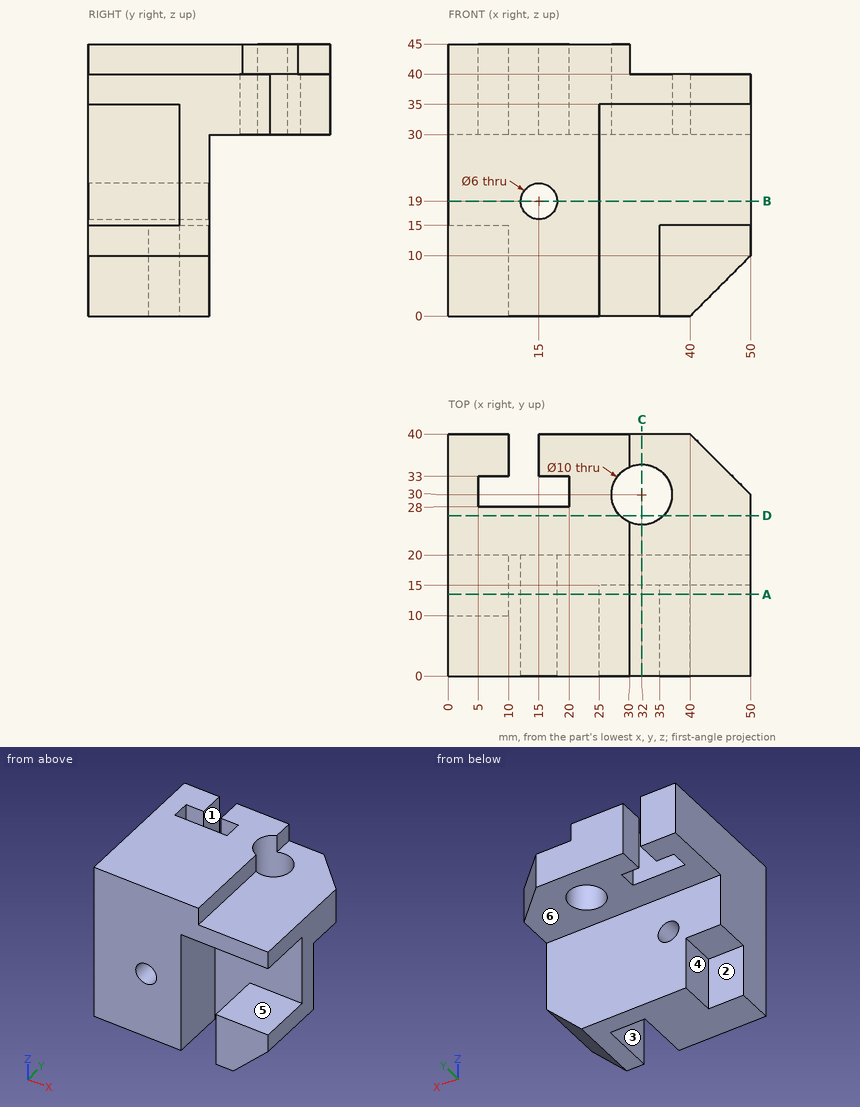
Geometry check sheet. Reference: drawing and pictorial views, mm from the part's lowest x, y, z. A direction names the side the tool comes from. Give positions to 0.01 mm unless a question says otherwise; leave off trailing zeros. Order: outer loops, then holes, each group sorted by start corner. A loop starts at its lowest first (then second) coordinate and runs counter-clockwise, first axis right, second up. Notation, with made-up numbers: M 59.25,-35.75 L 118.25,-35.75 A19 cw 118.25,-10.75 Z; hole C 65,-11 d6. An arc over 180 degrees is marked long. Answer in a Markdown table with one row per item. Add a question column.
Item 1: Mould release check, pull along Z, two halves, no side actions. Record for the marked faces 4, 5 and 6: released by +Z, released by -Z, zero draft, split by the parting line, or undercut.
Item 2: Scan lines: probe 1 along X at (y, z) = (5, 19); probe 2 along X at (y, z) = (30, 37.5); probe 3 along X at (y, z) = (30, 40.75). Record each from-to range of solid material in increasing order. Write a range as from..to.
Item 3: Section check B-B, the plane z = 19. Enter the section's corners in (x, y), and give its area (3 significant figures).
Item 4: Tool access check on the marked faces 1, 2 and 3. Record the directions out of +Z, -Z, +X, -X, +Y, -Y that give a thin tool (end or side, any length) a straight path to the whole face; none if there is none.
Item 5: Section check C-C, the plane x = 32. Enter the section's corners in (y, z), and give its area (3 significant figures).
Item 6: Gauge pin test, flat ends, axial feed: pin 1 (5 mm diameter, centred on x = 4, y = 15.5, fed in from -Z); pin 2 (1 mm diameter, centred on x = 11.5, z = 26.5, fed in from +Y); pin 3 (10 mm diameter, centred on x = 42, y = 29.5, fed in from +Z). Record the tip position at first contact, or that the pin passes through.
Item 7: Section check A-A, the plane y = 13.5. Enter the section's corners in (x, z).
Item 8: Section check D-D, the plane y = 26.5. Enter the section's corners in (x, z), and give its area (3 significant figures).
Filled sheet:
| question | item | result |
|---|---|---|
| 1 | face 4 | zero draft |
| 1 | face 5 | undercut |
| 1 | face 6 | released by -Z |
| 2 | probe 1 | x = 0..12, 18..25 |
| 2 | probe 2 | x = 0..5, 20..27, 37..50 |
| 2 | probe 3 | x = 0..5, 20..27 |
| 3 | outline | M 0,0 L 12,0 L 12,20 L 0,20 Z; M 18,0 L 25,0 L 25,15 L 50,15 L 50,20 L 18,20 Z |
| 3 | area | 505 mm^2 |
| 4 | face 1 | +Z, -Z, +Y |
| 4 | face 2 | -Z, -X, +Y |
| 4 | face 3 | -Z, -Y |
| 5 | outline | M 0,35 L 15,35 L 15,0 L 20,0 L 20,30 L 25,30 L 25,40 L 0,40 Z; M 35,30 L 40,30 L 40,40 L 35,40 Z |
| 5 | area | 375 mm^2 |
| 6 | pin 1 | stops at z = 15 |
| 6 | pin 2 | stops at y = 20 |
| 6 | pin 3 | stops at z = 40 |
| 7 | outline | M 0,15 L 10,15 L 10,0 L 25,0 L 25,35 L 50,35 L 50,40 L 30,40 L 30,45 L 0,45 Z; M 35,0 L 40,0 L 50,10 L 50,15 L 35,15 Z; hole C 15,19 d6 |
| 8 | outline | M 0,30 L 28.43,30 L 28.43,45 L 0,45 Z; M 35.57,30 L 50,30 L 50,40 L 35.57,40 Z |
| 8 | area | 571 mm^2 |
